from build123d import *

# Parameters (mm, degrees)
SKETCH_3_R = 1.4


with BuildPart() as part:
    # 扫描1: sweep along a path in 草图2
    with BuildLine(Plane.XY) as sweep_1_path:
        Line((-22.258775921, 79.972270587), (-20.392109255, 75.333784243))
        ThreePointArc((-20.392109255, 75.333784243), (-20.701297553, 44.720670994), (-42.566666667, 23.292560165))
        Line((-42.566666667, 23.292560165), (-79.674557412, 8.359226832))
    # 草图3 → 扫描1 (sweep)
    with BuildSketch(Plane(origin=(-79.674557412, 8.359226832, 0), x_dir=(0, 0, 1), z_dir=(-0.9276972686292776, -0.3733333333333338, 0))):
        Circle(SKETCH_3_R)
    sweep(path=sweep_1_path.line)

    # 草图4 → 旋转1 (revolve)
    with BuildSketch(Plane(origin=(-65.674557412, -26.429420742, 0), x_dir=(0, 0, 1), z_dir=(-0.9276972686292776, -0.37333333333333385, 0))):
        with BuildLine():
            Line((0, 38.9), (0, 36.1))
            ThreePointArc((0, 36.1), (-1.4, 37.5), (0, 38.9))
        make_face()
    revolve(axis=Axis((-80.197224079, 9.658003008, 0), (0.37333333333333635, -0.9276972686292765, 0)))

    # 草图6 → 旋转2 (revolve)
    with BuildSketch(Plane(origin=(-30.8, 76.535024662, 0), x_dir=(0.9276972686292776, 0.37333333333333374, 0), z_dir=(-0.3733333333333337, 0.9276972686292775, 0))):
        with BuildLine():
            Line((7.806908727, 0), (10.606908727, 0))
            ThreePointArc((10.606908727, 0), (9.206908727, 1.4), (7.806908727, 0))
        make_face()
    revolve(axis=Axis((-23.557552098, 79.44960392, 0), (0.9276972686292784, 0.3733333333333317, 0)))


solid = part.part
Source: CAD feature listing. Evaluate the final solid. Frame: model axes, mm. Coordinates: 2 decimals unless noted, no trailing zeros. Loops run counter-clockwise (first coordinate to the right, second up) from the corner with the lowest first, then second, coordinate; pieces in that order, holes last. Notation, with made-up numbers: (23.5, 24) - (47.5, 24) arc R15 ccw to (47.5, 39) - close; hole circle Ø1 at (32.5, 6.5). An arc over 180 degrees is marked (long way). One line per item, written item: value. Start each with the question number.
1. Contact query for a flat-ended pin moving along its axis: P1, Ø1.5, axis at y = 71, z = -1, coming from the -X side. Output: stop coordinate, or through.
2. Ray query, L1, parallel to Y at x = -22, z = -0.05; L2, parallel to X at y = 65, z = 0.75; L3, parallel to Y at x = -57, z = -0.4. Return the intervals inside material, ascending.
3. Section A-A (z = 0.45). Return the cut outline in (x, y).
4. Mould query, pull axis Y, two halves, no side actions, for faces 1 (the cylindrical face through (-20.16, 78.08, 0.65)), 2 (the cylindrical face through (-61.82, 16.82, 0.75)). Classes: pulls with the +Y half, pulls with the -Y half, needs draft (parallel to the pull), parting line crosses it, or undercut.
Verdict:
1. P1: stops at x = -20.46
2. L1: y = 39.1 to 45.24, 75.58 to 81.35
2. L2: x = -18.96 to -16.58
2. L3: y = 16.04 to 18.93
3. outline: (-80.17, 9.59) arc R1.33 ccw to (-79.18, 7.13) - (-42.07, 22.06) arc R41.33 ccw to (-19.16, 75.83) - (-21.03, 80.47) arc R1.33 ccw to (-23.49, 79.48) - (-21.62, 74.84) arc R38.67 cw to (-43.06, 24.52) - close
4. face 1: undercut
4. face 2: parting line crosses it
